from build123d import *

# Parameters (mm, degrees)
SCHIZZO1_W                      = 30
SCHIZZO1_H                      = 30
SCHIZZO1_R                      = 6
ESTRUSIONE_ESTRUSIONE1_DEPTH    = 30
F_8_0_8_DIAMETER_HOLE1_D        = 8
F_8_0_8_DIAMETER_HOLE1_DEPTH    = 13.5
F_8_0_8_DIAMETER_HOLE1_TIP      = 2.403442476
FORO_FILETTATO_M3_1_AT_2_COUNT  = 2
FORO_FILETTATO_M3_1_AT_2_PITCH  = 20
FORO_FILETTATO_M3_2_D           = 2.5
FORO_FILETTATO_M3_2_DEPTH       = 8.5
FORO_FILETTATO_M3_2_CSINK_D     = 3.05
FORO_FILETTATO_M3_2_CSINK_ANGLE = 120
FORO_FILETTATO_M3_2_TIP         = 0.751075774
CHAMFER1_SIZE                   = 0.5
CHAMFER2_SIZE                   = 0.2


with BuildPart() as part:
    # Schizzo1 → Estrusione-Estrusione1 (new body)
    with BuildSketch(Plane.XY):
        with Locations((15, 15)):
            Rectangle(SCHIZZO1_W, SCHIZZO1_H)
        with Locations((12, 16.8)):
            Circle(SCHIZZO1_R, mode=Mode.SUBTRACT)
    extrude(amount=ESTRUSIONE_ESTRUSIONE1_DEPTH)

    # Ø8.0 (8) Diameter Hole1
    with Locations(Plane(origin=(30, 0, 0), x_dir=(0, 0, -1), z_dir=(1, 0, 0))):
        with Locations((-15, 10)):
            Hole(F_8_0_8_DIAMETER_HOLE1_D / 2, depth=F_8_0_8_DIAMETER_HOLE1_DEPTH)
            with Locations((0, 0, -(F_8_0_8_DIAMETER_HOLE1_DEPTH + F_8_0_8_DIAMETER_HOLE1_TIP / 2))):  # 118° drill point
                Cone(0, F_8_0_8_DIAMETER_HOLE1_D / 2, F_8_0_8_DIAMETER_HOLE1_TIP, mode=Mode.SUBTRACT)

    # Schizzo7 → Foro filettato M3-1 (revolve, cut)
    with BuildSketch(Plane(origin=(5, 30, 25), x_dir=(0, 0, 1), z_dir=(1, 0, 0))):
        Polygon((0, 0), (0, 9.251075774), (1.25, 8.5), (1.25, 0.158771324), (1.525, 0), align=None)
    foro_filettato_m3_1 = revolve(axis=Axis((5, 36.35, 25), (0, -1, 0)), mode=Mode.SUBTRACT)

    # Foro filettato M3-1 at 2: Foro filettato M3-1 ×2
    with Locations(*[(i * FORO_FILETTATO_M3_1_AT_2_PITCH, 0, 0) for i in range(1, FORO_FILETTATO_M3_1_AT_2_COUNT)]):
        add(foro_filettato_m3_1, mode=Mode.SUBTRACT)

    # Specchia1: Foro filettato M3-1 across plane
    add(foro_filettato_m3_1.mirror(Plane.XY.offset(15)), mode=Mode.SUBTRACT)

    # Specchia1 copy 1 sketch → Specchia1 copy 1 (revolve, cut)
    with BuildSketch(Plane(origin=(25, 30, 5), x_dir=(0, 0, -1), z_dir=(1, 0, 0))):
        Polygon((0, 0), (0, -9.251075774), (1.25, -8.5), (1.25, -0.158771324), (1.525, 0), align=None)
    revolve(axis=Axis((25, 36.35, 5), (0, 1, 0)), mode=Mode.SUBTRACT)

    # Foro filettato M3-2
    with Locations(Plane(origin=(0, 0, 0), x_dir=(-1, 0, 0), z_dir=(0, -1, 0))):
        with Locations((-27, -15)):
            CounterSinkHole(FORO_FILETTATO_M3_2_D / 2, FORO_FILETTATO_M3_2_CSINK_D / 2, depth=FORO_FILETTATO_M3_2_DEPTH, counter_sink_angle=FORO_FILETTATO_M3_2_CSINK_ANGLE)
            with Locations((0, 0, -(FORO_FILETTATO_M3_2_DEPTH + FORO_FILETTATO_M3_2_TIP / 2))):  # 118° drill point
                Cone(0, FORO_FILETTATO_M3_2_D / 2, FORO_FILETTATO_M3_2_TIP, mode=Mode.SUBTRACT)

    # Chamfer1
    chamfer1_edges = [part.edges().sort_by_distance(p)[0] for p in [
        (30, 15, 30),
        (15, 30, 30),
        (0, 15, 30),
        (15, 30, 0),
        (30, 15, 0),
        (15, 0, 0),
        (0, 15, 0),
        (15, 0, 30),
        (0, 30, 15),
        (30, 30, 15),
        (30, 0, 15),
        (0, 0, 15),
    ]]
    chamfer(chamfer1_edges, length=CHAMFER1_SIZE)

    # Chamfer2
    chamfer2_edges = [part.edges().sort_by_distance(p)[0] for p in [
        (6, 16.8, 0),
        (6, 16.8, 30),
        (30, 10, 11),
    ]]
    chamfer(chamfer2_edges, length=CHAMFER2_SIZE)


solid = part.part
Could you check a few things on this model? Use its own coordinates, in mm. A direction names the side the tool comes from. Give positions to 0.01 mm unless a question says otherwise; leave off trailing zeros. Order: outer loops, then holes, each group sorted by start corner. A loop starts at its lowest first (then second) coordinate and runs counter-clockwise, first axis right, second up.
Item 1: If we section it at D-D, the plane x = 27: Write out the boundary of the cut face in (y, z) (3 decimals), plus the area to 3 significant figures.
Item 2: For faces 5 (the face through (26.22, 25.73, 5.27)), 6 (the face through (23.057, 11.201, 18.815)), 7 (the face through (14.769, 11.477, 14.793)), which set-ups out of +Z, -Z, +X, -X, +Y, -Y let a thin tool reach every point of the face, with its end or its side?
Item 3: I'm going to push flat-ended pins straight in: pin 1 (6.5 mm diameter, centred on y = 10, z = 15, fed in from +X); pin 2 (5 mm diameter, centred on x = 14, y = 18.5, fed in from +Z); pin 3 (15.5 mm diameter, centred on x = 12, y = 16.8, fed in from +Z). Where does each tip first touch, or does it pass through?
Item 4: If we mould it in two halves opening along Z, with no side actions, what happens to faces 1 (the face through (18, 12, 30)), 2 (the face through (6.22, 25.73, 5.27)), 3 (the face through (27.672, 3.222, 13.946)), 4 (the face through (30, 15, 15))? For each: pulls with the +Z half, pulls with the -Z half, needs draft (parallel to the pull), parting line crosses it, or undercut.
Item 5: If we section it at A-A, the plane y = 16.8: Write out the boundary of the cut face in (x, z).
Item 6: If we section it at B-B, the plane x = 12: Write out the boundary of the cut face in (y, z), plus the area to 3 significant figures.
Item 7: I need wall thicknesses on line 1 (Z direction, x = 25, y = 25); line 2 (Z direction, x = 27, y = 3.5). Which ranges of each line are inside material? Lowest first, please.
Item 8: If we section it at C-C, the plane z = 21: Write out the boundary of the cut face in (x, y).
Values:
1. outline: (0, 0.5) - (0.5, 0) - (29.5, 0) - (30, 0.5) - (30, 29.5) - (29.5, 30) - (0.5, 30) - (0, 29.5) - (0, 16.525) - (0.159, 16.25) - (6.2, 16.25) arc R4 cw (long way) to (6.2, 13.75) - (0.159, 13.75) - (0, 13.475) - close
1. area: 834 mm2
2. face 5: +Y
2. face 6: +X
2. face 7: +Z, -Z
3. pin 1: stops at x = 16.05
3. pin 2: passes through
3. pin 3: stops at z = 30
4. face 1: pulls with the +Z half
4. face 2: undercut
4. face 3: undercut
4. face 4: needs draft
5. outline: (0, 0.5) - (0.5, 0) - (5.8, 0) - (6, 0.2) - (6, 29.8) - (5.8, 30) - (0.5, 30) - (0, 29.5) - close; (18, 0.2) - (18.2, 0) - (29.5, 0) - (30, 0.5) - (30, 29.5) - (29.5, 30) - (18.2, 30) - (18, 29.8) - close
6. outline: (0, 0.5) - (0.5, 0) - (10.6, 0) - (10.8, 0.2) - (10.8, 29.8) - (10.6, 30) - (0.5, 30) - (0, 29.5) - close; (22.8, 0.2) - (23, 0) - (29.5, 0) - (30, 0.5) - (30, 29.5) - (29.5, 30) - (23, 30) - (22.8, 29.8) - close
6. area: 539 mm2
7. line 1: z = 0 to 3.75, 6.25 to 23.75, 26.25 to 30
7. line 2: z = 0 to 13.75, 16.25 to 30
8. outline: (0, 0.5) - (0.5, 0) - (29.5, 0) - (30, 0.5) - (30, 29.5) - (29.5, 30) - (0.5, 30) - (0, 29.5) - close; hole circle Ø12 at (12, 16.8)
